Autodesk Inventor part; units mm, degrees
ref_plane "XZ Plane" through (0, 0, 0) normal (0, 1, 0) x (-1, 0, 0)
ref_plane "XY Plane" through (0, 0, 0) normal (0, 0, 1) x (1, 0, 0)
sketch "Sketch1" plane through (0, 0, 0) normal (0, 0, 1) x (1, 0, 0)
  line L0 (-52.5, -17.5) -> (52.5, -17.5)
  line L1 (52.5, -17.5) -> (52.5, 17.5)
  line L2 (52.5, 17.5) -> (-52.5, 17.5)
  line L3 (-52.5, 17.5) -> (-52.5, -17.5)
  line L4 (-52.5, -17.5) -> (52.5, 17.5) construction
  line L5 (52.5, -17.5) -> (-52.5, 17.5) construction
  point P0 (0, 0)
  dimension "d0" = 105
  dimension "d1" = 35
extrude "Extrusion1" add sketch "Sketch1" along normal blind 20
sketch "Sketch2" plane through (0, 0, 20) normal (0, 0, 1) x (1, 0, 0)
  line L0 (52.5, 17.5) -> (-52.5, 17.5)
  line L1 (-42.5, 17.5) -> (42.5, 17.5)
  line L2 (42.5, 17.5) -> (42.5, -7.5)
  line L3 (42.5, -7.5) -> (-42.5, -7.5)
  line L4 (-42.5, -7.5) -> (-42.5, 17.5)
  line L5 (-52.5, 17.5) -> (-52.5, -17.5)
  line L6 (52.5, -17.5) -> (52.5, 17.5)
  line L7 (-52.5, -17.5) -> (52.5, -17.5)
  point P0 (0, 0)
  point P1 (42.5, 17.5)
  dimension "d4" = 10
  dimension "d5" = 10
  dimension "d6" = 10
extrude "Extrusion2" cut sketch "Sketch2" against normal through all contours L2 L3 L4 L0
chamfer "Chamfer1" distance 20 angle 45 2 edges at (-42.5, -7.5, 10) (42.5, -7.5, 10)
fillet "Fillet1" radius 2 4 edges at (-42.5, 12.5, 10) (-22.5, -7.5, 10) (22.5, -7.5, 10) (42.5, 12.5, 10)
sketch "Sketch3" plane through (-21.6716, -7.5, 20) normal (0, 1, 0) x (1, 0, 0)
  line L0 (-35.2748, 10) -> (83.1656, 10) construction
  circle A0 centre (-0.3284, 10) radius 2.5
  line L1 (21.6716, 24) -> (21.6716, -4)
  circle A1 centre (43.6716, 10) radius 2.5
  point P0 (21.6716, 20)
  dimension "d13" = 5
  dimension "d14" = 22
extrude "Extrusion3" cut sketch "Sketch3" against normal through all both and the other way through all
sketch "Sketch4" plane through (-21.6716, -7.5, 20) normal (0, 1, 0) x (1, 0, 0)
  arc A0 (-1.4142, 12.2519) -> (-1.4142, 7.7481) centre (-0.3284, 10) ccw
  arc A1 (44.7574, 7.7481) -> (44.7574, 12.2519) centre (43.6716, 10) ccw
  circle A2 centre (-0.3284, 10) radius 5.5
  circle A3 centre (43.6716, 10) radius 5.5
  point P0 (21.6716, 20)
  dimension "d17" = 11
  dimension "d18" = 11
extrude "Extrusion4" cut sketch "Sketch4" along normal blind 20
sketch "Sketch5" plane through (52.5, -17.5, 0) normal (1, 0, 0) x (0, 0, -1)
  circle A0 centre (-10, 23) radius 2.5
  line L0 (-20, 0) -> (-20, 35)
  line L1 (0, 35) -> (-20, 35)
  point P0 (0, 17.5)
  dimension "d21" = 10
  dimension "d22" = 12
  dimension "d23" = 5
extrude "Extrusion5" cut sketch "Sketch5" against normal through all
chamfer "Chamfer2" distance 2 angle 45 6 edges at (-52.5, 0, 20) (-52.5, 0, 0) (52.5, 0, 20) (52.5, 0, 0) (-52.5, -17.5, 10) (52.5, -17.5, 10)
sketch "Sketch6" plane through (-42.5, 17.5, 20) normal (1, 0, 0) x (0, 0, -1)
  circle A0 centre (10, -12) radius 2.5
  circle A1 centre (10, -12) radius 5.5
  point P0 (20, -17.5)
  dimension "d29" = 11
extrude "Extrusion6" cut sketch "Sketch6" along normal blind 20
mirror "Mirror1" about plane through (0, 0, 0) normal (1, 0, 0) of "Extrusion6"
sketch "Sketch7" plane through (-42.5, 5.5, 10) normal (1, 0, 0) x (0, 0, -1)
  circle A0 centre (0, 0) radius 5.5
  line L0 (4.0415, 0) -> (2.0207, -3.5)
  line L1 (2.0207, -3.5) -> (-2.0207, -3.5)
  line L2 (-2.0207, -3.5) -> (-4.0415, 0)
  line L3 (-4.0415, 0) -> (-2.0207, 3.5)
  line L4 (-2.0207, 3.5) -> (2.0207, 3.5)
  line L5 (2.0207, 3.5) -> (4.0415, 0)
  point P0 (10, -5.5)
  dimension "d32" = 7
extrude "Extrusion7" add sketch "Sketch7" along normal up to surface surface through (-32.5, 2.5, 20) normal (0.7071, 0.7071, 0)
sketch "Sketch8" plane through (-21.6716, -7.5, 20) normal (0, 1, 0) x (1, 0, 0)
  arc A0 (-1.4142, 15.3918) -> (-1.4142, 4.6082) centre (-0.3284, 10) ccw
  circle A1 centre (-0.3284, 10) radius 5.5
  line L0 (-0.3284, 14.0415) -> (3.1716, 12.0207)
  line L1 (3.1716, 12.0207) -> (3.1716, 7.9793)
  line L2 (3.1716, 7.9793) -> (-0.3284, 5.9585)
  line L3 (-0.3284, 5.9585) -> (-3.8284, 7.9793)
  line L4 (-3.8284, 7.9793) -> (-3.8284, 12.0207)
  line L5 (-3.8284, 12.0207) -> (-0.3284, 14.0415)
  point P0 (21.6716, 20)
  dimension "d35" = 7
extrude "Extrusion8" cut sketch "Sketch8" against normal blind 4 contours L0 L1 L2 L3 L4 L5
mirror "Mirror2" about plane through (0, 0, 0) normal (1, 0, 0) of "Extrusion7", "Extrusion8"
properties part number "_3DPrint"
Geometry check sheet. Reference: the model listing, model coordinates, mm. A direction names the side the tool comes from. Round coordinates to 2 decimals unless told otherwise and drop trailing zeros. Loops run counter-clockwise (first coordinate to the right, second up) from the corner with the lowest first, then second, coordinate; pieces in that order, holes last. Notation, with made-up numbers: (7.25, 61) -> (52.25, 61) arc R16 cw to (52.25, 86) -> close; hole circle Ø2 at (54, 53.5). An arc over 180 degrees is marked (long way). Use a Markdown table: item, result.
(1) Sectioned sample at C-C (y = -12.5). Enter the section's corners in (x, z).
Calculated:
| item | result |
|---|---|
| outline | (-52.5, 2) -> (-50.5, 0) -> (50.5, 0) -> (52.5, 2) -> (52.5, 18) -> (50.5, 20) -> (-50.5, 20) -> (-52.5, 18) -> close; hole circle Ø5 at (-22, 10); hole circle Ø5 at (22, 10) |
(2) Sectioned sample at A-A (y = 14.5). Enter the section's corners in (x, z).
Calculated:
| item | result |
|---|---|
| outline | (-52.5, 2) -> (-50.5, 0) -> (-42.5, 0) -> (-42.5, 20) -> (-50.5, 20) -> (-52.5, 18) -> close; (42.5, 0) -> (50.5, 0) -> (52.5, 2) -> (52.5, 18) -> (50.5, 20) -> (42.5, 20) -> close |
(3) Mould release check, pull along Y, two halves, no side actions. Record for faces 4 (the flat face through (23.725, -9.472, 6.955)), 5 (the flat face through (-47, 17.5, 10)), 6 (the flat face through (38.49, 3.774, 13.045)): released by +Y, released by -Y, zero draft, split by the parting line, or undercut.
Calculated:
| item | result |
|---|---|
| face 4 | zero draft |
| face 5 | released by +Y |
| face 6 | undercut |
(4) Sectioned sample at B-B (x = 45.5). Enter the section's corners in (y, z).
Calculated:
| item | result |
|---|---|
| outline | (-17.5, 0) -> (17.5, 0) -> (17.5, 20) -> (-17.5, 20) -> close; hole circle Ø5 at (5.5, 10) |
(5) Scan lines: probe 1 along X at (y, z) = (-15.2, 10); probe 2 along Y at (x, z) = (-50, 10); probe 3 along X at (y, z) = (-2.5, 10.75). Record each from-to range of solid material in increasing order.
Calculated:
| item | result |
|---|---|
| probe 1 | -52.5 to -24.5, -19.5 to 19.5, 24.5 to 52.5 |
| probe 2 | -17.5 to 3, 8 to 17.5 |
| probe 3 | -52.5 to -27.5, 27.5 to 52.5 |
(6) Sectioned sample at D-D (z = 10). Give the number of separate pieces and of enclosed holes in the cut face, then the cut area to 3 significant figures.
Calculated:
| item | result |
|---|---|
| separate pieces | 5 |
| enclosed holes | 0 |
| area | 1,610 mm² |
(7) Set-up check for faces 1 (the flat face through (22, -11.5, 13)), 2 (the flat face through (-42.5, 15, 10)), 3 (the flat face through (-38.49, 3.775, 6.955)): record each of +Z, -Z, +X, -X, +Y, -Y from which the full face is reachable in a straight line by a thin tool's end or side.
Calculated:
| item | result |
|---|---|
| face 1 | +Y |
| face 2 | +Z, -Z, +Y |
| face 3 | none |
(8) Go/stop test with flat-tipped pins: P1, Ø6.5, axis at y = 5.5, z = 10, coming from the +X side; P2, Ø10, axis at x = 11, z = 8.5, coming from the +Y side; P3, Ø1.2, axis at x = -37.5, z = 10.5, coming from the +Y side; P4, Ø1, axis at x = -27.5, z = 6.5, coming from the +Y side. Record where each tip stops, or that it passes through.
Calculated:
| item | result |
|---|---|
| P1 | x = 52.5 |
| P2 | y = -7.5 |
| P3 | y = 2 |
| P4 | y = -2 |
